Design review of the part shown in the three views and the two pictorial views. Dimensions are in mm from the part's minimum x, y and z. A direction names the side the tool comes from. Give positions to 0.01 mm unless a question says otherwise; leave off trailing zeros. Write each loop counter-clockwise with the first axis right and the second up, starting at its lowest first coordinate (ties: lowest second). Pieces come first, ordered by that corner, then holes. Notation, with made-up numbers: M -33.5,59 L -2.5,59 A20 cw -2.5,67 Z; hole C -27.5,17 d2. An arc over 180 degrees is marked long. Use one line per item in the form item = value. Start each with the question number.
Q1. Clearance check with flat-ended pins moving along their axes: pin 1 Ø5 at (x, y) = (6.5, 7.5) entering from +Z; pin 2 Ø6 at (x, z) = (5.5, 3) entering from +Y; pin 3 Ø6 at (x, y) = (17.5, 3.5) entering from +Z; pin 4 Ø5 at (y, z) = (9.5, 14) entering from +X. State where each tip first meets the part, or that it passes through.
Q2. Mouldability with a two-part tool opening along Z and no side actions: class the marked faces 1, 2 and 3 as released by +Z, released by -Z, zero draft, split by the parting line, or undercut.
Q3. Tool access review of the marked faces 4 and 5: name each direction out of +Z, -Z, +X, -X, +Y, -Y from which nothing blocks a thin tool from reaching the whole face with its end or side.
Q4. Consider section A-A on z = 8. Write out the cut boundary in (x, y).
Q5. Consider section C-C on y = 1.5. Write out the cut boundary in (x, z).
Q6. For probe 1 along Z at (x, y) = (10, 4.5); probe 2 along X at (y, z) = (3.25, 8); probe 3 along Z at (x, y) = (10.5, 10), list the stretches that pass through material, from the lowest coordinate up. Write a range as [from, to].
Q7. Consider section B-B on y = 11.75. Write out the cut boundary in (x, z), and give its area (3 significant figures).
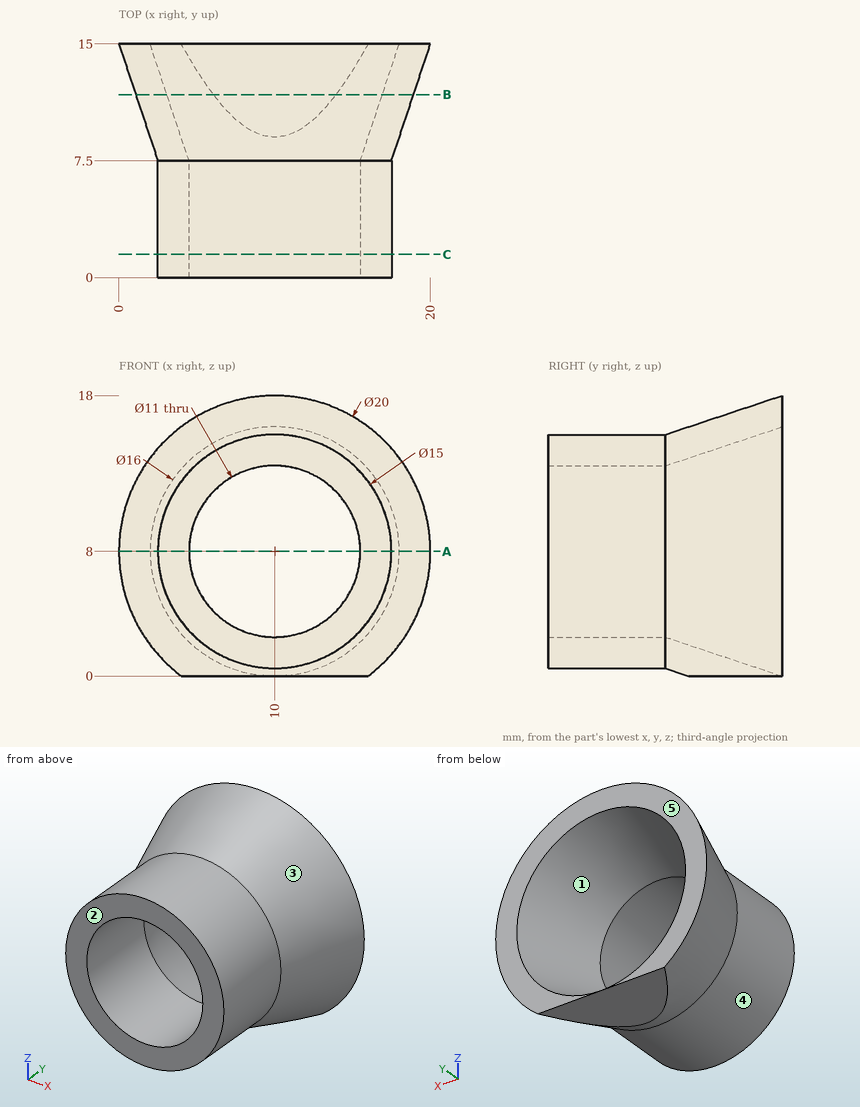
Working result:
q1.pin_1 = 15.92
q1.pin_2 = 15
q1.pin_3 = 14
q1.pin_4 = 17.69
q2.face_1 = undercut
q2.face_2 = zero draft
q2.face_3 = split by the parting line
q3.face_4 = -Y
q3.face_5 = +Z, -Z, +X, -X, +Y
q4.outline = M 0,15 L 2.5,7.5 L 2.5,0 L 4.5,0 L 4.5,7.5 L 2,15 Z; M 15.5,0 L 17.5,0 L 17.5,7.5 L 20,15 L 18,15 L 15.5,7.5 Z
q5.outline = C 10,8 d15; hole C 10,8 d11
q6.probe_1 = [0.5, 2.5], [13.5, 15.5]
q6.probe_2 = [2.5, 4.5], [15.5, 17.5]
q6.probe_3 = [0, 1.69], [14.31, 16.32]
q7.outline = M 6.06,0 L 13.94,0 A8.92 ccw long Z; hole C 10,8 d13.83
q7.area = 94.6 mm²
